from build123d import *

# Parameters (mm, degrees)
SKETCH_1_W          = 58
SKETCH_1_H          = 50
EXTRUDE_1_DEPTH     = 10
SKETCH_2_R          = 29
SKETCH_2_R_2        = 26.1
EXTRUDE_2_DEPTH     = 7.5
SKETCH_3_R          = 26.1
SKETCH_3_R_2        = 24
EXTRUDE_3_DEPTH     = 0.5
CUT_EXTRUDE_1_REACH = 12
SKETCH_5_R          = 1.55
SKETCH_6_R          = 3
CUT_EXTRUDE_2_DEPTH = 3
SKETCH_7_R          = 15
CUT_EXTRUDE_3_DEPTH = 11


with BuildPart() as part:
    # 草图1 → 凸台-拉伸1 (new body)
    with BuildSketch(Plane.XY):
        with BuildLine():
            ThreePointArc((-29, 25), (0, 54), (29, 25))
            Line((29, 25), (-29, 25))
        make_face()
        Rectangle(SKETCH_1_W, SKETCH_1_H)
    extrude(amount=EXTRUDE_1_DEPTH)

    # 草图2 → 凸台-拉伸2 (add)
    with BuildSketch(Plane(origin=(0, 0, 0), x_dir=(-1, 0, 0), z_dir=(0, 0, -1))):
        with Locations((0, 25)):
            Circle(SKETCH_2_R)
        with Locations((0, 25)):
            Circle(SKETCH_2_R_2, mode=Mode.SUBTRACT)
    extrude(amount=EXTRUDE_2_DEPTH)

    # 草图3 → 凸台-拉伸3 (add)
    with BuildSketch(Plane(origin=(0, 0, 0), x_dir=(-1, 0, 0), z_dir=(0, 0, -1))):
        with Locations((0, 25)):
            Circle(SKETCH_3_R)
        with Locations((0, 25)):
            Circle(SKETCH_3_R_2, mode=Mode.SUBTRACT)
    extrude(amount=EXTRUDE_3_DEPTH)

    # 草图5 → 切除-拉伸1 (cut, up to next)
    with BuildSketch(Plane(origin=(0, 0, 0), x_dir=(-1, 0, 0), z_dir=(0, 0, -1)), mode=Mode.PRIVATE) as cut_extrude_1_sk1:
        with Locations((-19, -20)):
            Circle(SKETCH_5_R)
    cut_extrude_1_tool1 = extrude(cut_extrude_1_sk1.sketch, amount=-CUT_EXTRUDE_1_REACH, mode=Mode.PRIVATE) & part.part
    add(cut_extrude_1_tool1.solids().sort_by_distance((19, -20, 0))[0], mode=Mode.SUBTRACT)
    # 草图5 → 切除-拉伸1 (cut, up to next)
    with BuildSketch(Plane(origin=(0, 0, 0), x_dir=(-1, 0, 0), z_dir=(0, 0, -1)), mode=Mode.PRIVATE) as cut_extrude_1_sk2:
        with Locations((-9, -20)):
            Circle(SKETCH_5_R)
    cut_extrude_1_tool2 = extrude(cut_extrude_1_sk2.sketch, amount=-CUT_EXTRUDE_1_REACH, mode=Mode.PRIVATE) & part.part
    add(cut_extrude_1_tool2.solids().sort_by_distance((9, -20, 0))[0], mode=Mode.SUBTRACT)
    # 草图5 → 切除-拉伸1 (cut, up to next)
    with BuildSketch(Plane(origin=(0, 0, 0), x_dir=(-1, 0, 0), z_dir=(0, 0, -1)), mode=Mode.PRIVATE) as cut_extrude_1_sk3:
        with Locations((9, -20)):
            Circle(SKETCH_5_R)
    cut_extrude_1_tool3 = extrude(cut_extrude_1_sk3.sketch, amount=-CUT_EXTRUDE_1_REACH, mode=Mode.PRIVATE) & part.part
    add(cut_extrude_1_tool3.solids().sort_by_distance((-9, -20, 0))[0], mode=Mode.SUBTRACT)
    # 草图5 → 切除-拉伸1 (cut, up to next)
    with BuildSketch(Plane(origin=(0, 0, 0), x_dir=(-1, 0, 0), z_dir=(0, 0, -1)), mode=Mode.PRIVATE) as cut_extrude_1_sk4:
        with Locations((19, -20)):
            Circle(SKETCH_5_R)
    cut_extrude_1_tool4 = extrude(cut_extrude_1_sk4.sketch, amount=-CUT_EXTRUDE_1_REACH, mode=Mode.PRIVATE) & part.part
    add(cut_extrude_1_tool4.solids().sort_by_distance((-19, -20, 0))[0], mode=Mode.SUBTRACT)

    # 草图6 → 切除-拉伸2 (cut)
    with BuildSketch(Plane.XY.offset(10)):
        with Locations((19, -20)):
            Circle(SKETCH_6_R)
        with Locations((9, -20)):
            Circle(SKETCH_6_R)
        with Locations((-9, -20)):
            Circle(SKETCH_6_R)
        with Locations((-19, -20)):
            Circle(SKETCH_6_R)
    extrude(amount=-CUT_EXTRUDE_2_DEPTH, mode=Mode.SUBTRACT)

    # 草图7 → 切除-拉伸3 (cut, through all)
    with BuildSketch(Plane(origin=(0, 0, 0), x_dir=(-1, 0, 0), z_dir=(0, 0, -1))):
        with Locations((0, 25)):
            Circle(SKETCH_7_R)
    extrude(amount=-CUT_EXTRUDE_3_DEPTH, mode=Mode.SUBTRACT)


solid = part.part
The listing builds one solid part. Answer for the finished solid, in the listing's coordinates (mm). A direction names the side the tool comes from. Coordinates: 2 decimals unless noted, no trailing zeros. Loops run counter-clockwise (first coordinate to the right, second up) from the corner with the lowest first, then second, coordinate; pieces in that order, holes last. Notation, with made-up numbers: M 35,-11.5 L 46,-11.5 A22 cw 46,10.5 Z; hole C 67,59.5 d6. An arc over 180 degrees is marked long. Answer in a Markdown table with one row per item.
1) Determine the mould class of faces 4 (the cylindrical face through (16.6, -21.8, 8.5)), 5 (the flat face through (0, -25, 5)), 6 (the flat face through (29, 0, 5)) for opening direction Y: released by +Y, released by -Y, zero draft, split by the parting line, or undercut.
Answers below:
| item | result |
|---|---|
| face 4 | undercut |
| face 5 | released by -Y |
| face 6 | zero draft |
2) Which of the six approach directions +Z, -Z, +X, -X, +Y, -Y give full straight-line access (tool end or side, diameter ignored) to faces 1 (the cylindrical face through (3.775, 53.753, -0.572)), 2 (the cylindrical face through (18.17, -18.69, 3.45)), 3 (the flat face through (-17.7, -21.3, 7))?
Answers below:
| item | result |
|---|---|
| face 1 | -Z |
| face 2 | +Z, -Z |
| face 3 | +Z |
3) Find section A-A (z = 8.75). Determine the outline of the cut face in (x, y).
Answers below:
| item | result |
|---|---|
| outline | M -29,-25 L 29,-25 L 29,25 A29 ccw -29,25 Z; hole C -19,-20 d6; hole C 0,25 d30; hole C -9,-20 d6; hole C 9,-20 d6; hole C 19,-20 d6 |
4) Find section B-B (x = -8.5). Determine the outline of the cut face in (y, z), then the cut area to 3 significant figures.
Answers below:
| item | result |
|---|---|
| outline | M -25,0 L -21.47,0 L -21.47,7 L -22.96,7 L -22.96,10 L -25,10 Z; M -18.53,0 L -2.73,0 L -2.73,-7.5 L 0.32,-7.5 L 0.32,-0.5 L 2.56,-0.5 L 2.56,0 L 12.64,0 L 12.64,10 L -17.04,10 L -17.04,7 L -18.53,7 Z; M 37.36,0 L 47.44,0 L 47.44,-0.5 L 49.68,-0.5 L 49.68,-7.5 L 52.73,-7.5 L 52.73,10 L 37.36,10 Z |
| area | 540 mm^2 |
5) Find section D-D (x = 14). Determine the outline of the cut face in (y, z), then the cut area to 3 significant figures.
Answers below:
| item | result |
|---|---|
| outline | M -25,0 L -0.4,0 L -0.4,-7.5 L 2.97,-7.5 L 2.97,-0.5 L 5.51,-0.5 L 5.51,0 L 19.61,0 L 19.61,10 L -25,10 Z; M 30.39,0 L 44.49,0 L 44.49,-0.5 L 47.03,-0.5 L 47.03,-7.5 L 50.4,-7.5 L 50.4,10 L 30.39,10 Z |
| area | 699 mm^2 |
6) Find the intervals of material crossed by probe 1 along Y at (x, z) = (0, -4); probe 2 along Y at (x, z) = (-9, 8.25); probe 3 along Y at (x, z) = (9, 2), in increasing order.
Answers below:
| item | result |
|---|---|
| probe 1 | -4 to -1.1, 51.1 to 54 |
| probe 2 | -25 to -23, -17 to 13, 37 to 52.57 |
| probe 3 | -25 to -21.55, -18.45 to 13, 37 to 52.57 |
7) Find section C-C (y = 31.5). Determine the outline of the cut face in (x, z).
Answers below:
| item | result |
|---|---|
| outline | M -28.26,-7.5 L -25.28,-7.5 L -25.28,-0.5 L -23.1,-0.5 L -23.1,0 L -13.52,0 L -13.52,10 L -28.26,10 Z; M 13.52,0 L 23.1,0 L 23.1,-0.5 L 25.28,-0.5 L 25.28,-7.5 L 28.26,-7.5 L 28.26,10 L 13.52,10 Z |
8) Given pin 1 (3 mm diameter, centred on x = -9, y = -21, fed in from +Z); pin 2 (15 mm diameter, centred on x = 0, y = 9.5, fed in from -Z); pin 3 (1.5 mm diameter, centred on y = 44, z = -5.5, fed in from +X), each flat-ended and moving along its own axis, determine where each tip first touches the part or whether it passes through.
Answers below:
| item | result |
|---|---|
| pin 1 | z = 7 |
| pin 2 | z = 0 |
| pin 3 | x = 22.54 |
